Check sheet for the modelled part. Datum: model origin and axes. Units: mm. A direction names the side the tool comes from. Give positions to 0.01 mm unless a question says otherwise; leave off trailing zeros. Order: outer loops, then holes, each group sorted by start corner. A loop starts at its lowest first (then second) coordinate and runs counter-clockwise, first axis right, second up.
```python
from build123d import *

# Parameters (mm, degrees)
SKIZZE1_W                       = 300
SKIZZE1_H                       = 75
LINEAR_AUSTRAGEN1_DEPTH         = 10
SCHNITT_LINEAR_AUSTRAGEN1_DEPTH = 10
VERRUNDUNG1_R                   = 3


with BuildPart() as part:
    # Skizze1 → Linear austragen1 (new body)
    with BuildSketch(Plane.XY):
        with Locations((0, -112.5)):
            Rectangle(SKIZZE1_W, SKIZZE1_H)
    extrude(amount=LINEAR_AUSTRAGEN1_DEPTH)

    # Skizze2 → Schnitt-Linear austragen1 (cut)
    with BuildSketch(Plane.XY.offset(10)):
        Polygon((-34, -140), (34, -140), (34, -136), (50, -136), (50, -84), (34, -84), (34, -80), (-34, -80), (-34, -84), (-50, -84), (-50, -136), (-34, -136), align=None)
    extrude(amount=-SCHNITT_LINEAR_AUSTRAGEN1_DEPTH, mode=Mode.SUBTRACT)

    # Verrundung1
    verrundung1_edges = [part.edges().sort_by_distance(p)[0] for p in [
        (-34, -140, 5),
        (-50, -136, 5),
        (-50, -84, 5),
        (-34, -80, 5),
        (34, -80, 5),
        (50, -84, 5),
        (50, -136, 5),
        (34, -140, 5),
    ]]
    fillet(verrundung1_edges, radius=VERRUNDUNG1_R)


solid = part.part
```
(1) Tool access check on faces 1 (the face through (41, -84, 5)), 2 (the face through (-150, -113, 5)). Record the directions out of +Z, -Z, +X, -X, +Y, -Y that give a thin tool (end or side, any length) a straight path to the whole face; none if there is none.
(2) Thickness scan on L1, parallel to X at y = -129.5, z = 4.25; L2, parallel to Y at x = 4, z = 4; L3, parallel to X at y = -139.5, z = 7.75. Record the ranges inside material, lowest first.
(3) Sectioned sample at B-B (y = -111.5). Enter the section's corners in (x, z), plus the area to 3 significant figures.
(4) Sectioned sample at A-A (x = 16.5). Enter the section's corners in (y, z), plus the area to 3 significant figures.
(5) Release check for a two-part mould opening along X. For faces 3 (the face through (150, -113, 5)), 4 (the face through (-2, -145, 10)), 5 (the face through (-41, -136, 5)) record: released by +X, released by -X, zero draft, split by the parting line, or undercut.
(6) Sectioned sample at C-C (z = 4.25). Enter the section's corners in (x, y).
Values follow:
1. face 1: +Z, -Z
1. face 2: +Z, -Z, -X, +Y, -Y
2. L1: x = -150 to -50, 50 to 150
2. L2: y = -150 to -140, -80 to -75
2. L3: x = -150 to -32.66, 32.66 to 150
3. outline: (-150, 0) - (-50, 0) - (-50, 10) - (-150, 10) - close; (50, 0) - (150, 0) - (150, 10) - (50, 10) - close
3. area: 2,000 mm2
4. outline: (-150, 0) - (-140, 0) - (-140, 10) - (-150, 10) - close; (-80, 0) - (-75, 0) - (-75, 10) - (-80, 10) - close
4. area: 150 mm2
5. face 3: released by +X
5. face 4: zero draft
5. face 5: undercut
6. outline: (-150, -150) - (150, -150) - (150, -75) - (-150, -75) - close; hole (-50, -133) arc R3 ccw to (-47, -136) - (-34, -136) - (-34, -137) arc R3 ccw to (-31, -140) - (31, -140) arc R3 ccw to (34, -137) - (34, -136) - (47, -136) arc R3 ccw to (50, -133) - (50, -87) arc R3 ccw to (47, -84) - (34, -84) - (34, -83) arc R3 ccw to (31, -80) - (-31, -80) arc R3 ccw to (-34, -83) - (-34, -84) - (-47, -84) arc R3 ccw to (-50, -87) - close
